Source: CAD feature listing. Evaluate the final solid. Frame: model axes, mm. Face numbers are marked on the shaded views. Give positions to 0.01 mm unless a question says otherwise; leave off trailing zeros. Loops run counter-clockwise (first coordinate to the right, second up) from the corner with the lowest first, then second, coordinate; pieces in that order, holes last.
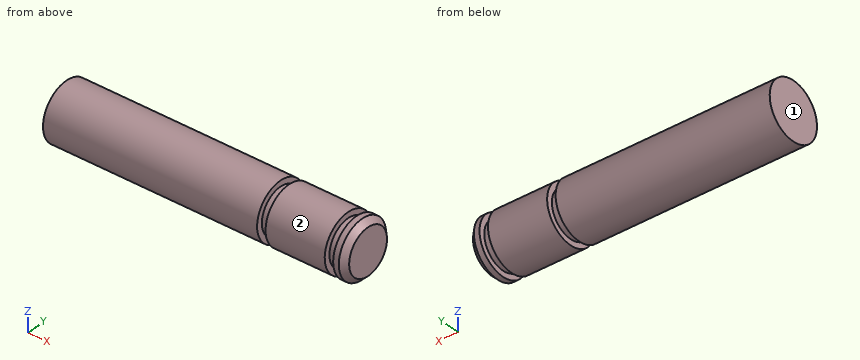
from build123d import *

# Parameters (mm, degrees)
CHAMFER1_SIZE = 1


with BuildPart() as part:
    # Sketch1 → Revolve1 (revolve)
    with BuildSketch(Plane.XY, mode=Mode.PRIVATE) as revolve1_sk:
        Polygon((0, 0), (0, 5), (38, 5), (38, 4), (39.5, 4), (39.5, 5), (50, 5), (50, 4), (51.5, 4), (51.5, 5), (53.5, 5), (53.5, 0), align=None)
    revolve(revolve1_sk.sketch.rotate(Axis((-16.67807852, 0, 0), (1, 0, 0)), 90), axis=Axis((-16.67807852, 0, 0), (1, 0, 0)))

    # Chamfer1
    chamfer1_edges = [part.edges().sort_by_distance(p)[0] for p in [
        (53.5, 0, -5),
    ]]
    chamfer(chamfer1_edges, length=CHAMFER1_SIZE)


solid = part.part
1) Ray query, probe 1 along X at (y, z) = (-2, 4); probe 2 along X at (y, z) = (1.75, 4); probe 3 along Z at (x, y) = (2, -3). Return the intervals inside material, ascending.
Checks:
probe 1: x = 0 to 38, 39.5 to 50, 51.5 to 53.03
probe 2: x = 0 to 38, 39.5 to 50, 51.5 to 53.13
probe 3: z = -4 to 4
2) Contact query for flat-ended pins moving along their axis: P1, Ø4, axis at x = 19.5, y = 3, coming from the -Z side; P2, Ø1, axis at x = 9.5, z = 1, coming from the -Y side; P3, Ø4, axis at x = 11.5, z = -3, coming from the +Y side. Output: stop coordinate, or through.
Checks:
P1: stops at z = -4.9
P2: stops at y = -4.97
P3: stops at y = 4.9
3) Pull-direction query (Y, two-part tool) for the marked faces 1 and 2; classes: released by +Y, released by -Y, zero draft, split by the parting line, or undercut.
Checks:
face 1: zero draft
face 2: split by the parting line
4) Cut plane A-A (x = 36.5). Return loops of the section in (y, z).
Checks:
outline: circle Ø10 at (0, 0)
